Job drawing, mm, ordinate dimensions from the low corner. One solid piece. A direction names the side the tool comes from. Give positions to 0.01 mm unless a question says otherwise; leave off trailing zeros. Write each loop counter-clockwise with the first axis right and the second up, starting at its lowest first coordinate (ties: lowest second). Pieces come first, ordered by that corner, then holes. Notation, with made-up numbers: M 39,-7 L 82,-7 A20 ccw 82,27 Z; hole C 55.5,39 d3. An arc over 180 degrees is marked long. Use CSV: the item, a comma, the result in double quotes. Start each with the question number.
Item 1: Cut at D-D (x = 17.5). List the corners of the cut face in (y, z) (3 decimals), then the cut area to 3 significant figures.
Item 2: Cut at A-A (x = 25.4). List the corners of the cut face in (y, z) (3 decimals), then the cut area to 3 significant figures.
Item 3: Mould opens along X. For the marked faces 3, 4, 5 and 6 say: released by +X, released by -X, zero draft, split by the parting line, or undercut.
Item 4: Cut at B-B (z = 12.7). List the corners of the cut face in (x, y) (3 decimals).
Item 5: Cut at C-C (y = 13.5). List the corners of the cut face in (x, z) (3 decimals).
Item 6: Which spindle directions (+Z, -Z, +X, -X, +Y, -Y) get a long thin tool onto all of the face, cutting with end or side? Do the marked faces 1 and 2. Say none if no direction does.
Item 7: Drill centre lines: line 1 (Y direction, x = 4.5, z = 73) (3 decimals); line 2 (X direction, y = 5.75, z = 83.5) (3 decimals); line 3 (X direction, y = 0.95, z = 12.7). Where is each one in solid material? Low to high. Write a range as [from, to].
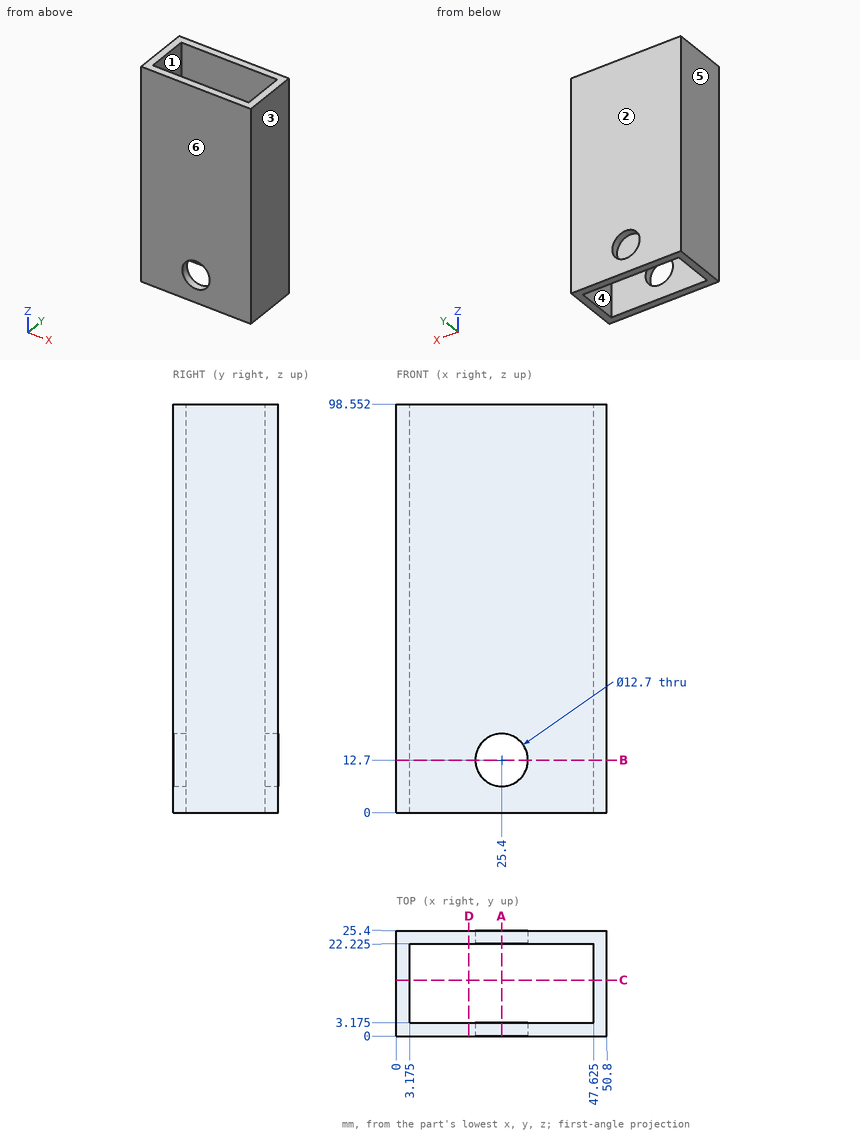
Worked answers:
1,outline,"M 0,0 L 3.175,0 L 3.175,98.552 L 0,98.552 Z; M 22.225,0 L 25.4,0 L 25.4,98.552 L 22.225,98.552 Z"
1,area,"626 mm^2"
2,outline,"M 0,0 L 3.175,0 L 3.175,6.35 L 0,6.35 Z; M 0,19.05 L 3.175,19.05 L 3.175,98.552 L 0,98.552 Z; M 22.225,0 L 25.4,0 L 25.4,6.35 L 22.225,6.35 Z; M 22.225,19.05 L 25.4,19.05 L 25.4,98.552 L 22.225,98.552 Z"
2,area,"545 mm^2"
3,face 3,"released by +X"
3,face 4,"undercut"
3,face 5,"released by -X"
3,face 6,"zero draft"
4,outline,"M 0,0 L 19.05,0 L 19.05,3.175 L 3.175,3.175 L 3.175,22.225 L 19.05,22.225 L 19.05,25.4 L 0,25.4 Z; M 31.75,0 L 50.8,0 L 50.8,25.4 L 31.75,25.4 L 31.75,22.225 L 47.625,22.225 L 47.625,3.175 L 31.75,3.175 Z"
5,outline,"M 0,0 L 3.175,0 L 3.175,98.552 L 0,98.552 Z; M 47.625,0 L 50.8,0 L 50.8,98.552 L 47.625,98.552 Z"
6,face 1,"+Z, -Z"
6,face 2,"+Z, -Z, +X, -X, +Y"
7,line 1,"y = [0, 3.175], [22.225, 25.4]"
7,line 2,"x = [0, 3.175], [47.625, 50.8]"
7,line 3,"x = [0, 19.05], [31.75, 50.8]"
